Work out the finished part from the listing and answer in its coordinate system (mm). A direction names the side the tool comes from. Round coordinates to 2 decimals unless told otherwise and drop trailing zeros. Order: outer loops, then holes, each group sorted by start corner. A loop starts at its lowest first (then second) coordinate and runs counter-clockwise, first axis right, second up. Notation, with made-up numbers: (-8, -10.75) - (13, -10.75) arc R9 ccw to (13, 0.25) - close; hole circle Ø4 at (24.25, 6). An arc over 180 degrees is marked (long way). Put each result on its own line as item: value.
```python
from build123d import *

# Parameters (mm, degrees)
F1_DEPTH = 19.05
F2_R     = 6.35
F3_DEPTH = 88.9
F4_SIZE  = 1.27


with BuildPart() as f1:
    # F0 (on Front) → F1 (new body)
    with BuildSketch(Plane.XZ):
        Polygon((3.178722, 10.529161), (-7.529159, 8.017435), (-10.707882, -2.511726), (-3.178722, -10.529161), (7.529159, -8.017435), (10.707882, 2.511726), align=None)
    extrude(amount=-F1_DEPTH)

    # F2 (on Front) → F3 (join)
    with BuildSketch(Plane.XZ):
        Circle(F2_R)
    extrude(amount=F3_DEPTH)

    # F4
    f4_edges = [f1.edges().sort_by_distance(p)[0] for p in [
        (-6.35, -88.9, 0),
        (-9.118521, 19.05, 2.752854),
        (-2.175218, 19.05, 9.273298),
        (-6.943302, 19.05, -6.520443),
        (2.175218, 19.05, -9.273298),
        (9.118521, 19.05, -2.752854),
        (6.943302, 19.05, 6.520443),
    ]]
    chamfer(f4_edges, length=F4_SIZE)


solid = f1.part
```
1) Given pin 1 Ø3 at (x, y) = (6, -13.5) entering from +Z; pin 2 Ø12 at (y, z) = (-34, -7) entering from +X; pin 3 Ø6 at (x, y) = (1.5, 2) entering from -Z, each flat-ended and moving along its own axis, determine where each tip first touches the part or whether it passes through.
Findings below:
pin 1: stops at z = 4.48
pin 2: stops at x = 6.27
pin 3: stops at z = -10.14
2) A cutting plane is placed at B-B on y = -28. Write down the section's boundary in (x, z), then the cut area to 3 significant figures.
Findings below:
outline: circle Ø12.7 at (0, 0)
area: 127 mm2
3) Straight lines are drawn through the part: L1, parallel to Y at x = -3.75, z = -7.25; L2, parallel to Y at x = -1, z = -5; L3, parallel to X at y = -12.5, z = -0.5. For each, find the intervals that lie inside material, in ascending order. Write a range as from..to.
Findings below:
L1: y = 0..19.05
L2: y = -88.88..19.05
L3: x = -6.33..6.33
4) A cutting plane is placed at A-A on z = 0. Write down the section's boundary in (x, y).
Findings below:
outline: (-9.95, 0) - (-6.35, 0) - (-6.35, -87.63) - (-5.08, -88.9) - (5.08, -88.9) - (6.35, -87.63) - (6.35, 0) - (9.95, 0) - (9.95, 17.78) - (8.62, 19.05) - (-8.62, 19.05) - (-9.95, 17.78) - close
5) For faces 1 (the flat face through (5, 0, -5)), 2 (the flat face through (2.1, 8.77, -9.29)), determine the directions among +Z, -Z, +X, -X, +Y, -Y from which every point of the face is accessible in a straight line to the end or side of a thin tool.
Findings below:
face 1: -Y
face 2: -Z, +X, +Y, -Y
6) A cutting plane is placed at C-C on x = 0. Write down the section's boundary in (y, z), then the cut area to 3 significant figures.
Findings below:
outline: (-88.9, -5.08) - (-87.63, -6.35) - (0, -6.35) - (0, -9.78) - (17.78, -9.78) - (19.05, -8.48) - (19.05, 8.48) - (17.78, 9.78) - (0, 9.78) - (0, 6.35) - (-87.63, 6.35) - (-88.9, 5.08) - close
area: 1,500 mm2
